Work out the finished part from the listing and answer in its coordinate system (mm). Face numbers are marked on the shaded views. A direction names the side the tool comes from. Round coordinates to 2 decimals unless told otherwise and drop trailing zeros. Loops run counter-clockwise (first coordinate to the right, second up) from the corner with the lowest first, then second, coordinate; pieces in that order, holes last.
from build123d import *

# Parameters (mm, degrees)
F0_W     = 127
F0_H     = 63.5
F1_DEPTH = 38.1
F2_W     = 101.6
F2_H     = 12.7
F3_DEPTH = 63.5
F4_W     = 38.1
F4_H     = 12.7
F5_DEPTH = 127.001
F7_D     = 19.05


with BuildPart() as f1:
    # F0 (on Top) → F1 (new body)
    with BuildSketch(Plane.XY):
        with Locations((-13.469666, -27.621665)):
            Rectangle(F0_W, F0_H)
    extrude(amount=F1_DEPTH)

    # F2 (on face) → F3 (cut, through all)
    with BuildSketch(Plane.XZ.offset(59.371665)):
        with Locations((-13.469666, 31.75)):
            Rectangle(F2_W, F2_H)
    extrude(amount=-F3_DEPTH, mode=Mode.SUBTRACT)

    # F4 (on face) → F5 (cut, through all)
    with BuildSketch(Plane.YZ.offset(50.030334)):
        with Locations((-27.556809, 6.35)):
            Rectangle(F4_W, F4_H)
    extrude(amount=-F5_DEPTH, mode=Mode.SUBTRACT)

    # F7 (through all)
    with Locations(Plane.XY.offset(25.4)):
        with Locations((-35.552364, -27.488971), (2.547636, -27.488971)):
            Hole(F7_D / 2)


solid = f1.part
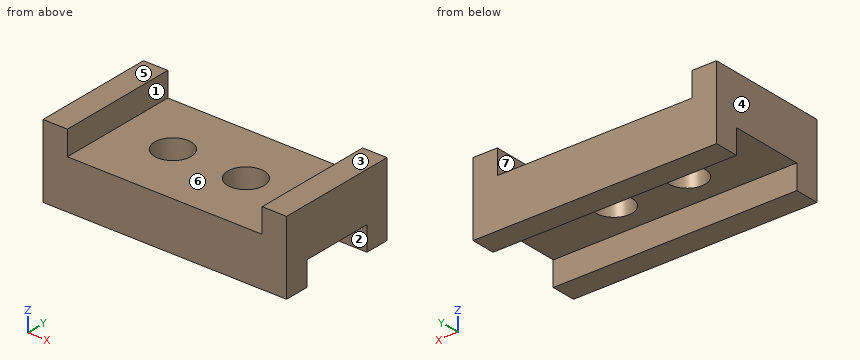
Item 1: Section C-C, the plane y = -25 is taken. Give the vertices of the cut face in (x, z), plus the area to 3 significant figures.
Item 2: Section B-B, the plane x = -36.5 is taken. Give the vertices of the cut face in (y, z), plus the area to 3 significant figures.
Item 3: Section A-A, the plane z = 35.5 is taken. Give the vertices of the cut face in (x, y).
Item 4: Each of these flat-tipped pins is pushed along its axis until it touches: P1, Ø8, axis at x = 21.5, y = -34, coming from the -Z side; P2, Ø12, axis at x = -51.5, y = -46, coming from the +Z side; P3, Ø5, axis at y = -14, z = 12.5, coming from the +X side. Where does it stop, or does it pass through?
Item 5: Straight lines are drawn through the part: line 1 (X direction, y = -13, z = 29); line 2 (Y direction, x = -8.5, z = 11.5); line 3 (Z direction, x = -5.5, y = -54.5). For each, find the intervals that lie inside material, in ascending order.
Item 6: Section D-D, the plane x = -59 is taken. Give the vertices of the cut face in (y, z).
Item 7: Determine the mould class of the marked faces 4, 5, 6 and 7 for opening direction X: pulls with the +X half, pulls with the -X half, needs draft (parallel to the pull), parting line crosses it, or undercut.
Item 8: For the marked faces 1, 2 and 3, determine the directions among +Z, -Z, +X, -X, +Y, -Y from which every point of the face is accessible in a straight line to the end or side of a thin tool.
Answer below:
1. outline: (-76.97, 12.7) - (-44.75, 12.7) - (-44.75, 25.4) - (-64.27, 25.4) - (-64.27, 38.1) - (-76.97, 38.1) - close; (-26.36, 12.7) - (-6.65, 12.7) - (-6.65, 25.4) - (-26.36, 25.4) - close; (11.74, 12.7) - (50.03, 12.7) - (50.03, 38.1) - (37.33, 38.1) - (37.33, 25.4) - (11.74, 25.4) - close
1. area: 1,470 mm2
2. outline: (-59.37, 0) - (-46.61, 0) - (-46.61, 12.7) - (-36.97, 12.7) - (-36.97, 25.4) - (-59.37, 25.4) - close; (-18.01, 12.7) - (-8.51, 12.7) - (-8.51, 0) - (4.13, 0) - (4.13, 25.4) - (-18.01, 25.4) - close
2. area: 888 mm2
3. outline: (-76.97, -59.37) - (-64.27, -59.37) - (-64.27, 4.13) - (-76.97, 4.13) - close; (37.33, -59.37) - (50.03, -59.37) - (50.03, 4.13) - (37.33, 4.13) - close
4. P1: stops at z = 12.7
4. P2: stops at z = 25.4
4. P3: stops at x = 50.03
5. line 1: x = -76.97 to -64.27, 37.33 to 50.03
5. line 2: y = -59.37 to -46.61, -8.51 to 4.13
5. line 3: z = 0 to 25.4
6. outline: (-59.37, 0) - (-46.61, 0) - (-46.61, 12.7) - (-8.51, 12.7) - (-8.51, 0) - (4.13, 0) - (4.13, 25.4) - (-59.37, 25.4) - close
7. face 4: pulls with the -X half
7. face 5: needs draft
7. face 6: undercut
7. face 7: undercut
8. face 1: +Z, +Y, -Y
8. face 2: -Z, +X, -X
8. face 3: +Z, +X, -X, +Y, -Y
